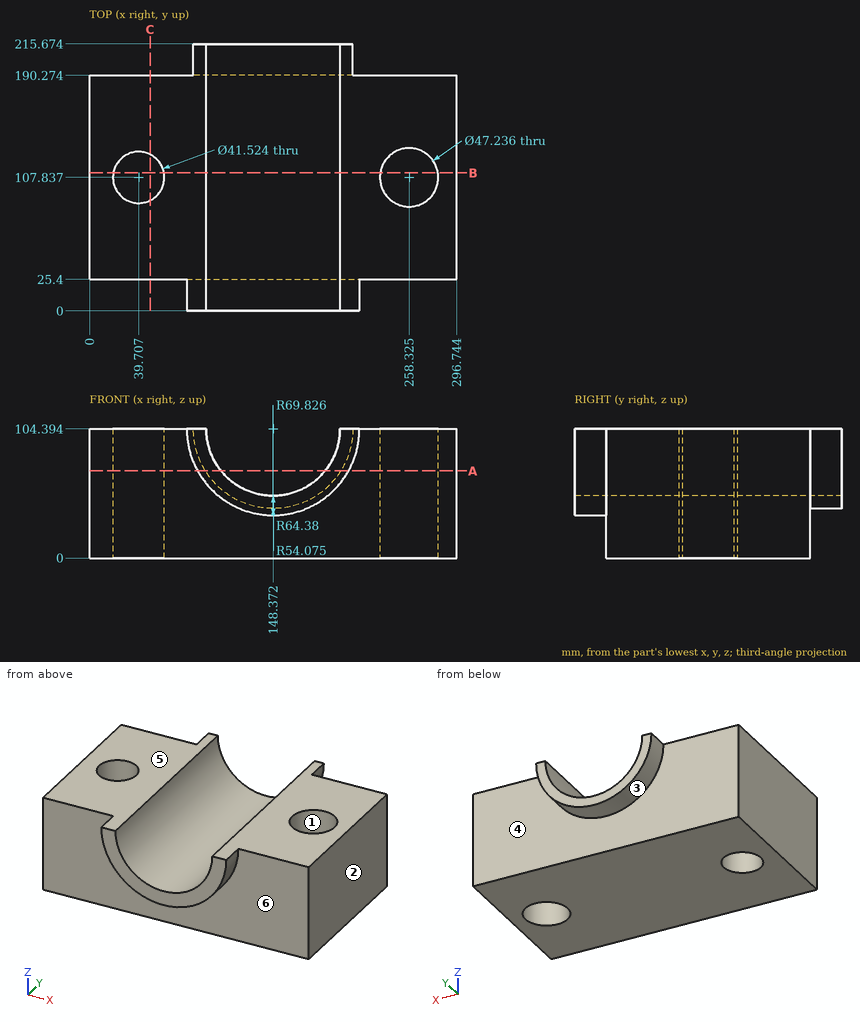
Verification items for this drawing (mm, ordinates from the low corner). A direction names the side the tool comes from. Give positions to 0.01 mm unless a question says otherwise; leave off trailing zeros. Loops run counter-clockwise (first coordinate to the right, second up) from the corner with the lowest first, then second, coordinate; pieces in that order, holes last. Notation, with made-up numbers: M 65,41.5 L 72,41.5 A30 cw 72,65.5 Z; hole C 63.25,57 d10. An arc over 180 degrees is marked long. Answer in a Markdown table with one row per item.
1) Cross-section at A-A (z = 70.5). Enter the section's corners in (x, y) (1 decimal), plus the area to 3 significant figures.
Solutions:
| item | result |
|---|---|
| outline | M 0,25.4 L 87.3,25.4 L 87.3,0 L 106.2,0 L 106.2,215.7 L 93.6,215.7 L 93.6,190.3 L 0,190.3 Z; M 190.5,0 L 209.4,0 L 209.4,25.4 L 296.7,25.4 L 296.7,190.3 L 203.1,190.3 L 203.1,215.7 L 190.5,215.7 Z; hole C 39.7,107.8 d41.5; hole C 258.3,107.8 d47.2 |
| area | 33,500 mm^2 |
2) Tool access check on the marked faces 4, 5 and 6. Record the directions out of +Z, -Z, +X, -X, +Y, -Y that give a thin tool (end or side, any length) a straight path to the whole face; none if there is none.
Solutions:
| item | result |
|---|---|
| face 4 | -Z, +Y |
| face 5 | +Z, +X, -X, +Y, -Y |
| face 6 | -Z, -Y |
3) Thickness scan on line 1 (X direction, y = 115, z = 57) (1 decimal); line 2 (X direction, y = 112, z = 99.5) (1 decimal); line 3 (X direction, y = 133.5, z = 71.5) (1 decimal). Record the ranges inside material, lowest first.
Solutions:
| item | result |
|---|---|
| line 1 | x = 0 to 20.2, 59.2 to 122.3, 174.4 to 235.8, 280.8 to 296.7 |
| line 2 | x = 0 to 19.4, 60 to 94.5, 202.2 to 235.1, 281.6 to 296.7 |
| line 3 | x = 0 to 105.5, 191.3 to 296.7 |
4) Cross-section at B-B (y = 111.5). Count the separate pieces of the cut face and the enclosed holes in it, plus the area to 3 significant figures.
Solutions:
| item | result |
|---|---|
| separate pieces | 3 |
| enclosed holes | 0 |
| area | 17,200 mm^2 |
5) Mould release check, pull along X, two halves, no side actions. Record for the marked faces 1, 2 and 3: released by +X, released by -X, zero draft, split by the parting line, or undercut.
Solutions:
| item | result |
|---|---|
| face 1 | undercut |
| face 2 | released by +X |
| face 3 | split by the parting line |
6) Cross-section at C-C (x = 49). Enter the section's corners in (y, z), plus the area to 3 significant figures.
Solutions:
| item | result |
|---|---|
| outline | M 25.4,0 L 89.27,0 L 89.27,104.39 L 25.4,104.39 Z; M 126.4,0 L 190.27,0 L 190.27,104.39 L 126.4,104.39 Z |
| area | 13,300 mm^2 |
7) Depth check by flat-ended pin: pin 1 (12 mm diameter, centred on x = 175, y = 70, fed in from +Z); pin 2 (5 mm diameter, centred on y = 22.5, z = 63.5, fed in from +X) (1 decimal). Enter the tip coordinate at first touch or a pass-through.
Solutions:
| item | result |
|---|---|
| pin 1 | stops at z = 61.27 |
| pin 2 | stops at x = 206.7 |
